```python
from build123d import *

# Parameters (mm, degrees)
F0_W      = 825.5
F0_H      = 723.9
F1_DEPTH  = 82.55
F2_W      = 711.2
F2_H      = 495.3
F3_DEPTH  = 82.55
F4_W      = 711.2
F4_H      = 66.675
F5_DEPTH  = 82.55
F6_W      = 711.2
F6_H      = 66.675
F7_DEPTH  = 82.55
F8_W      = 368.3
F8_H      = 82.55
F9_DEPTH  = 57.15
F10_R     = 6.985
F11_DEPTH = 762


with BuildPart() as f1:
    # F0 (on Top) → F1 (new body)
    with BuildSketch(Plane.XY):
        Rectangle(F0_W, F0_H)
    extrude(amount=F1_DEPTH)

    # F2 (on face) → F3 (cut)
    with BuildSketch(Plane.XY.offset(82.55)):
        Rectangle(F2_W, F2_H)
    extrude(amount=-F3_DEPTH, mode=Mode.SUBTRACT)

    # F4 (on face) → F5 (cut)
    with BuildSketch(Plane.XY.offset(82.55)):
        with Locations((0, 306.3875)):
            Rectangle(F4_W, F4_H)
    extrude(amount=-F5_DEPTH, mode=Mode.SUBTRACT)

    # F6 (on face) → F7 (cut)
    with BuildSketch(Plane.XY.offset(82.55)):
        with Locations((0, -306.3875)):
            Rectangle(F6_W, F6_H)
    extrude(amount=-F7_DEPTH, mode=Mode.SUBTRACT)

    # F8 (on face) → F9 (cut)
    with BuildSketch(Plane(origin=(-412.75, 0, 0), x_dir=(0, -1, 0), z_dir=(-1, 0, 0))):
        with Locations((0, 41.275)):
            Rectangle(F8_W, F8_H)
    extrude(amount=-F9_DEPTH, mode=Mode.SUBTRACT)

    # F10 (on face) → F11 (cut)
    with BuildSketch(Plane.XZ.offset(361.95)):
        with Locations((0, 32.385)):
            Circle(F10_R)
        with Locations((234.315, 32.385)):
            Circle(F10_R)
        with Locations((-234.315, 32.385)):
            Circle(F10_R)
    extrude(amount=-F11_DEPTH, mode=Mode.SUBTRACT)


solid = f1.part
```
Can you work these out from the model? Positions are in its coordinate system, mm. A direction names the side the tool comes from. Give positions to 0.01 mm unless a question says otherwise; leave off trailing zeros. Order: outer loops, then holes, each group sorted by start corner. A loop starts at its lowest first (then second) coordinate and runs counter-clockwise, first axis right, second up. Notation, with made-up numbers: M 34.25,13 L 63.25,13 A9 cw 63.25,30 Z; hole C 52,78.5 d11. An arc over 180 degrees is marked long. One line per item, written item: value.
1) For P1, Ø5, axis at y = 154.5, z = 52, coming from the -X side, with a flat end and sliding along its axis, tell me the tip position at first contact or that it passes through.
Answer sheet:
P1: stops at x = 355.6
2) I want a section at D-D, the plane y = -137.5. List the corners of the cut face in (x, z) for me.
Answer sheet:
outline: M 355.6,0 L 412.75,0 L 412.75,82.55 L 355.6,82.55 Z
3) Please list where these lines run through material, in increasing order: line 1 along Y through (x, z) = (-257, 17.5) (3 decimals); line 2 along Z through (x, y) = (0, 351.5).
Answer sheet:
line 1: y = -361.95 to -339.725, -273.05 to -247.65, 247.65 to 273.05, 339.725 to 361.95
line 2: z = 0 to 25.4, 39.37 to 82.55
4) I want a section at A-A, the plane y = 294. List the corners of the cut face in (x, z) for me.
Answer sheet:
outline: M -412.75,0 L -355.6,0 L -355.6,82.55 L -412.75,82.55 Z; M 355.6,0 L 412.75,0 L 412.75,82.55 L 355.6,82.55 Z
5) I want a section at B-B, the plane z = 10. List the corners of the cut face in (x, y) for me (3 decimals), plus the area to 3 significant figures.
Answer sheet:
outline: M -412.75,-361.95 L 412.75,-361.95 L 412.75,361.95 L -412.75,361.95 L -412.75,184.15 L -355.6,184.15 L -355.6,247.65 L 355.6,247.65 L 355.6,-247.65 L -355.6,-247.65 L -355.6,-184.15 L -412.75,-184.15 Z; hole M -355.6,-339.725 L 355.6,-339.725 L 355.6,-273.05 L -355.6,-273.05 Z; hole M -355.6,273.05 L 355.6,273.05 L 355.6,339.725 L -355.6,339.725 Z
area: 129,000 mm^2
6) On a 3-axis mill with a long thin cutter (end or side, diameter ignored), from which of +Z, -Z, +X, -X, +Y, -Y can I reach the whole of each face in a straight line? I mean faces 4 (the face through (-385, 184.15, 41)), 5 (the face through (355.6, 306, 42)), 6 (the face through (-412.75, -274, 41)). Say none if no direction works.
Answer sheet:
face 4: +Z, -Z, -X
face 5: +Z, -Z
face 6: +Z, -Z, -X, +Y, -Y
7) We'd pull the mould along Y, two halves only. Please class faces 1 (the face through (-355.6, -216, 42)), 2 (the face through (-6, -361.95, 41)), 3 (the face through (412.75, -5, 41)): released by +Y, released by -Y, zero draft, split by the parting line, or undercut.
Answer sheet:
face 1: undercut
face 2: released by -Y
face 3: zero draft
8) I want a section at C-C, the plane x = -254.5. List the corners of the cut face in (y, z) for me (3 decimals), plus the area to 3 significant figures.
Answer sheet:
outline: M -361.95,0 L -339.725,0 L -339.725,82.55 L -361.95,82.55 Z; M -273.05,0 L -247.65,0 L -247.65,82.55 L -273.05,82.55 Z; M 247.65,0 L 273.05,0 L 273.05,82.55 L 247.65,82.55 Z; M 339.725,0 L 361.95,0 L 361.95,82.55 L 339.725,82.55 Z
area: 7,860 mm^2
